Design review of the part built by this model. Coordinates are the model's own, in mm. A direction names the side the tool comes from. Give positions to 0.01 mm unless a question says otherwise; leave off trailing zeros. Write each loop counter-clockwise with the first axis right and the second up, starting at its lowest first coordinate (ties: lowest second). Pieces come first, ordered by that corner, then holes. Notation, with made-up numbers: (72, 65.5) - (96, 65.5) arc R32 cw to (96, 92.5) - close; hole circle Ø9 at (81, 46.25). An arc over 180 degrees is marked (long way). Write each question's results on one line, items separated by ' | '. Start each with the question number.
from build123d import *

# Parameters (mm, degrees)
SKETCH_W      = 100
SKETCH_H      = 100
SKETCH_R      = 1.5
PAD_DEPTH     = 2
SKETCH005_R   = 5
SKETCH005_R_2 = 1.5
PAD001_DEPTH  = 8.4
SKETCH007_W   = 4
SKETCH007_H   = 10
SKETCH007_W_2 = 3
SKETCH007_W_3 = 15
SKETCH007_H_2 = 3
SKETCH007_W_4 = 30
PAD002_DEPTH  = 8.4
POCKET_DEPTH  = 7.4


with BuildPart() as part:
    # Sketch → Pad (new body)
    with BuildSketch(Plane.XY):
        Rectangle(SKETCH_W, SKETCH_H)
        with Locations((-30, -30)):
            Circle(SKETCH_R, mode=Mode.SUBTRACT)
        with Locations((30, -30)):
            Circle(SKETCH_R, mode=Mode.SUBTRACT)
        with Locations((30, 30)):
            Circle(SKETCH_R, mode=Mode.SUBTRACT)
        with Locations((-30, 30)):
            Circle(SKETCH_R, mode=Mode.SUBTRACT)
        with Locations((-44, 44)):
            Circle(SKETCH_R, mode=Mode.SUBTRACT)
        with Locations((44, 44)):
            Circle(SKETCH_R, mode=Mode.SUBTRACT)
        with Locations((44, -44)):
            Circle(SKETCH_R, mode=Mode.SUBTRACT)
        with Locations((-44, -44)):
            Circle(SKETCH_R, mode=Mode.SUBTRACT)
    extrude(amount=PAD_DEPTH)

    # Sketch005 → Pad001 (join)
    with BuildSketch(Plane.XY.offset(2)):
        with Locations((-44, -44)):
            Circle(SKETCH005_R)
        with Locations((-44, -44)):
            Circle(SKETCH005_R_2, mode=Mode.SUBTRACT)
        with Locations((-44, 44)):
            Circle(SKETCH005_R)
        with Locations((-44, 44)):
            Circle(SKETCH005_R_2, mode=Mode.SUBTRACT)
        with Locations((44, 44)):
            Circle(SKETCH005_R)
        with Locations((44, 44)):
            Circle(SKETCH005_R_2, mode=Mode.SUBTRACT)
        with Locations((44, -44)):
            Circle(SKETCH005_R)
        with Locations((44, -44)):
            Circle(SKETCH005_R_2, mode=Mode.SUBTRACT)
    extrude(amount=PAD001_DEPTH)

    # Sketch007 → Pad002 (join)
    with BuildSketch(Plane.XY.offset(2)):
        with Locations((-3, -29)):
            Rectangle(SKETCH007_W, SKETCH007_H)
        with Locations((7.5, -33)):
            Rectangle(SKETCH007_W_2, SKETCH007_H)
        with Locations((0, -48.5)):
            Rectangle(SKETCH007_W_3, SKETCH007_H_2)
        with Locations((-26, -6.5)):
            Rectangle(SKETCH007_W_4, SKETCH007_H_2)
    extrude(amount=PAD002_DEPTH)

    # Sketch006 → Pocket (cut)
    with BuildSketch(Plane(origin=(0, 0, 0), x_dir=(1, 0, 0), z_dir=(0, 0, -1))):
        Polygon((-40.75, 44), (-42.375, 46.814583), (-45.625, 46.814583), (-47.25, 44), (-45.625, 41.185417), (-42.375, 41.185417), align=None)
        Polygon((45.625, 46.814583), (42.375, 46.814583), (40.75, 44), (42.375, 41.185417), (45.625, 41.185417), (47.25, 44), align=None)
        Polygon((45.625, -41.185417), (42.375, -41.185417), (40.75, -44), (42.375, -46.814583), (45.625, -46.814583), (47.25, -44), align=None)
        Polygon((-40.75, -44), (-42.375, -41.185417), (-45.625, -41.185417), (-47.25, -44), (-45.625, -46.814583), (-42.375, -46.814583), align=None)
    extrude(amount=-POCKET_DEPTH, mode=Mode.SUBTRACT)


solid = part.part
Q1. Add section D-D on z = 4.5. Count the separate pieces of the cut face and the enclosed holes in it, plus the area to 3 significant figures.
Q2. Machinability: for faces 1 (the face through (-7.5, -49, 6)), 2 (the face through (-5, -29, 6)), 3 (the face through (40, 47, 6)), 4 (the face through (-1, -29, 6)), 5 (the face through (-46.426, 42.573, 3.648)), which of the approach directions +Z, -Z, +X, -X, +Y, -Y give a long, thin tool a straight path to every point of the face, cutting with its end or side? Answer none if there is none.
Q3. The part is to be moulded in two halves that separate along Y. For faces 6 (the face through (-46.449, 45.388, 3.648)), 7 (the face through (-45.2, -42.8, 10.4)), say which applies: +Y half, -Y half, draft (parallel to the pull), parting line (faces both ways), or undercut.
Q4. For line 1 along Y through (x, z) = (-44, 8.55); line 2 along Y through (x, z) = (31, 1.5); line 3 along Y through (x, z) = (-18.5, 7.5), list the stretches that pass through material, from the lowest coordinate up. Write a range as [from, to].
Q5. Add section B-B on x = -44. State the section outline as (y, z) points.
Q6. Add section C-C on x = -14. State the section outline as (y, z) points, plus the area to 3 significant figures.
Q7. Insertion check: P1, Ø3.5, axis at x = -45, z = 2.5, coming from the +Y side; P2, Ø2.5, axis at x = -23.5, z = 5.5, coming from the +Y side; P3, Ø4, axis at y = -30.5, z = 5.5, coming from the +X side; P4, Ø2.5, axis at x = 7, z = 5.5, coming from the +Y side. Each pin has a flat end and moves straight along its axis. Give the tip position at first contact, or say it passes through.
Q8. Add section A-A on y = 30. State the section outline as (x, z) points.
Result:
1) separate pieces: 8 | enclosed holes: 4 | area: 409 mm²
2) face 1: +Z, +Y, -Y | face 2: +Z, -X, +Y | face 3: +Z | face 4: +Z, +Y | face 5: -Z
3) face 6: undercut | face 7: draft
4) line 1: y = [-49, -45.5], [-42.5, -39], [39, 42.5], [45.5, 49] | line 2: y = [-50, -31.12], [-28.88, 28.88], [31.12, 50] | line 3: y = [-8, -5]
5) outline: (-50, 0) - (-46.81, 0) - (-46.81, 7.4) - (-45.5, 7.4) - (-45.5, 10.4) - (-49, 10.4) - (-49, 2) - (-50, 2) - close; (-42.5, 7.4) - (-41.19, 7.4) - (-41.19, 0) - (41.19, 0) - (41.19, 7.4) - (42.5, 7.4) - (42.5, 10.4) - (39, 10.4) - (39, 2) - (-39, 2) - (-39, 10.4) - (-42.5, 10.4) - close; (45.5, 7.4) - (46.81, 7.4) - (46.81, 0) - (50, 0) - (50, 2) - (49, 2) - (49, 10.4) - (45.5, 10.4) - close
6) outline: (-50, 0) - (50, 0) - (50, 2) - (-5, 2) - (-5, 10.4) - (-8, 10.4) - (-8, 2) - (-50, 2) - close | area: 225 mm²
7) P1: stops at y = 50 | P2: stops at y = -5 | P3: stops at x = 9 | P4: stops at y = -28
8) outline: (-50, 0) - (-31.5, 0) - (-31.5, 2) - (-50, 2) - close; (-28.5, 0) - (28.5, 0) - (28.5, 2) - (-28.5, 2) - close; (31.5, 0) - (50, 0) - (50, 2) - (31.5, 2) - close
